Could you check a few things on this drawing? It's one solid part, dimensions in mm from its lowest x, y, z. A direction names the side the tool comes from. Give positions to 0.01 mm unless a question says otherwise; leave off trailing zeros. Order: outer loops, then holes, each group sorted by start corner. A loop starts at its lowest first (then second) coordinate and runs counter-clockwise, first axis right, second up.
(1) Will these pins go through, and if not, where does the flat tip stop? pin 1 (3 mm diameter, centred on y = 18.5, z = 12.5, fed in from -X); pin 2 (0.6 mm diameter, centred on x = 8, z = 11, fed in from -Y); pin 3 (10 mm diameter, centred on y = 19, z = 3, fed in from -X).
(2) Imagine slicing it at B-B, the plane x = 10. Write out the boundary of the cut face in (y, z), then the cut area to 3 significant figures.
(3) If I drill on probe 1 along Z at (x, y) = (10, 8); probe 2 along Y at (x, z) = (7.25, 5.75); probe 3 along Y at (x, z) = (14.75, 3.5), over which ranges is the centre line in solid material (lowest first)?
(4) If we mould it in two halves opening along X, with no side actions, what happens to the marked faces 1, 2 and 3? For each: released by +X, released by -X, zero draft, split by the parting line, or undercut.
(5) On a 3-axis mill with a long thin cutter (end or side, diameter ignored), from which of +Z, -Z, +X, -X, +Y, -Y can I reach the whole of each face in a straight line? I mean the marked faces 4 and 5. Say none if no direction works.
(6) Imagine slicing it at C-C, the plane y = 4.5. Write out the boundary of the cut face in (x, z).
(7) Imagine slicing it at A-A, the plane z = 10. Write out the boundary of the cut face in (x, y).
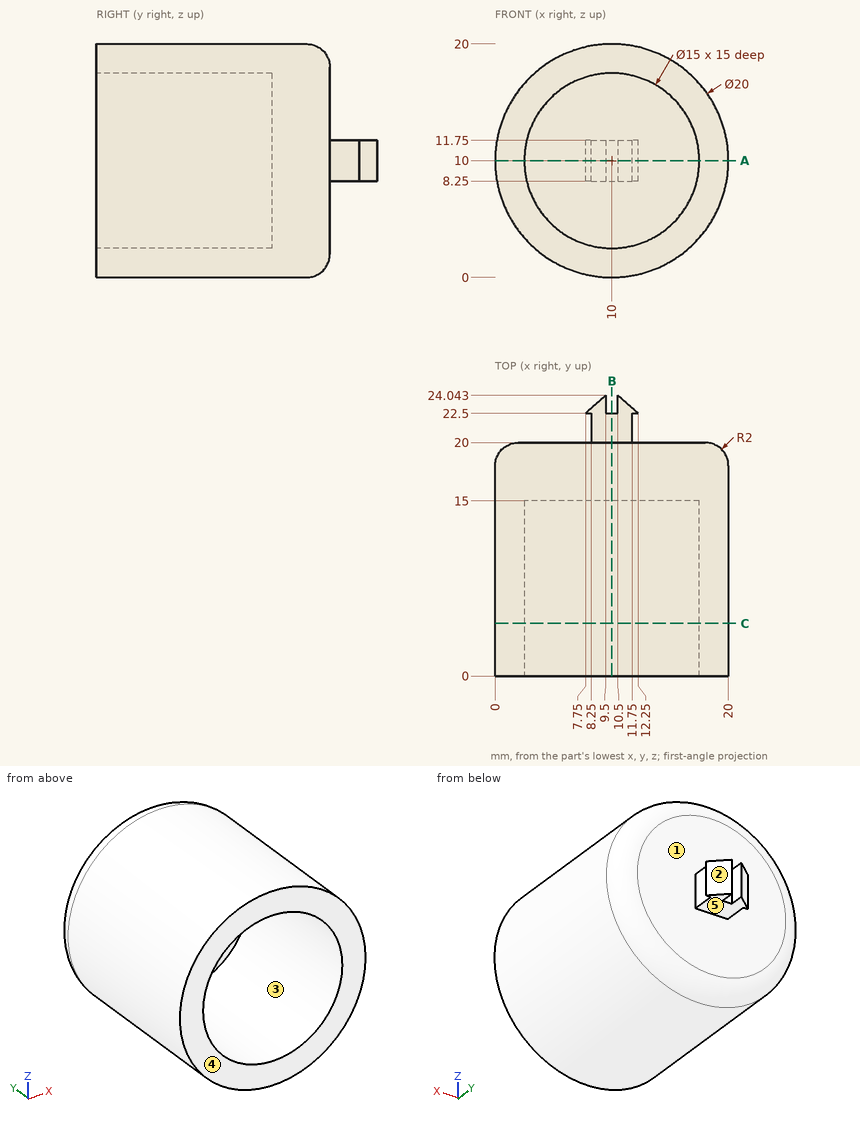
Answer block:
1. pin 1: stops at x = 0.06
1. pin 2: stops at y = 15
1. pin 3: stops at x = 0.22
2. outline: (0, 0) - (18, 0) arc R2 ccw to (20, 2) - (20, 8.25) - (22.5, 8.25) - (22.5, 11.75) - (20, 11.75) - (20, 18) arc R2 ccw to (18, 20) - (0, 20) - (0, 17.5) - (15, 17.5) - (15, 2.5) - (0, 2.5) - close
2. area: 182 mm2
3. probe 1: z = 0 to 2.5, 17.5 to 20
3. probe 2: y = 15 to 20
3. probe 3: y = 0 to 20
4. face 1: zero draft
4. face 2: released by +X
4. face 3: undercut
5. face 4: +Z, -Z, +X, -X, -Y
5. face 5: -Z, +X, -X, +Y
6. outline: circle Ø20 at (10, 10); hole circle Ø15 at (10, 10)
7. outline: (0, 0) - (2.5, 0) - (2.5, 15) - (17.5, 15) - (17.5, 0) - (20, 0) - (20, 18) arc R2 ccw to (18, 20) - (11.75, 20) - (11.75, 22.5) - (12.25, 22.5) - (10.5, 24.04) - (10.5, 22.5) - (9.5, 22.5) - (9.5, 24.04) - (7.75, 22.5) - (8.25, 22.5) - (8.25, 20) - (2, 20) arc R2 ccw to (0, 18) - close
